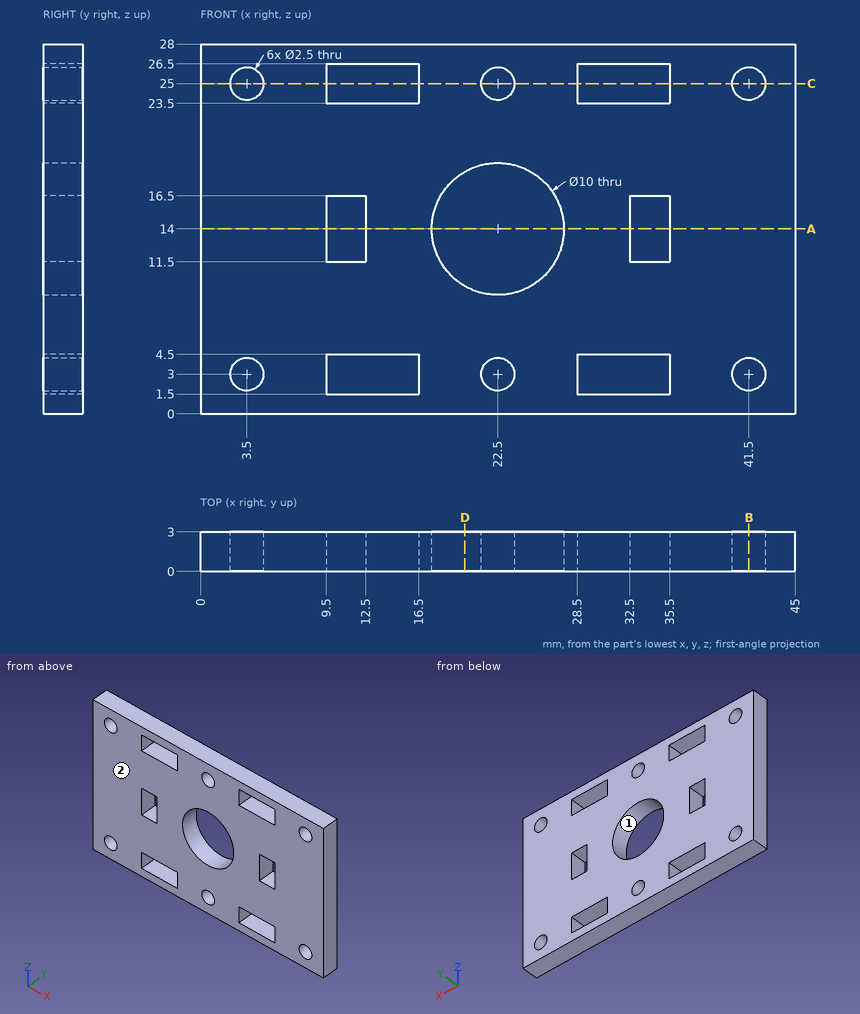
Check sheet for the drawn part. Datum: minimum x, y, z corner. Units: mm. Round coordinates to 2 decimals unless told otherwise and drop trailing zeros. Order: outer loops, then holes, each group sorted by start corner. A loop starts at its lowest first (then second) coordinate and runs counter-clockwise, first axis right, second up. Notation, with made-up numbers: (72, 38.5) -> (111, 38.5) arc R12 cw to (111, 49.5) -> close; hole circle Ø1 at (-22.75, 71.25). An arc over 180 degrees is marked (long way). Put each result on its own line as item: value. Start each with the question number.
(1) Draft check along Z on the marked faces 1 and 2. Enter one of: +Z half, -Z half, draft (parallel to the pull), parting line (faces both ways), or undercut.
(2) Depth check by flat-ended pin: pin 1 Ø3 at (x, z) = (37, 4) entering from -Y. Enter the tip coordinate at first touch or a pass-through.
(3) Section check C-C (z = 25). Enter the section's corners in (x, y), then the cut area to 3 significant figures.
(4) Section check D-D (x = 20). Enter the section's corners in (y, z), then the cut area to 3 significant figures.
(5) Material ranges on line 1 along X through (y, z) = (1.4, 25); line 2 along X through (y, z) = (1.4, 13.75); line 3 along Z through (x, y) = (22.5, 1.6), recorded low to high.
(6) Section check A-A (z = 14). Enter the section's corners in (x, y), then the cut area to 3 significant figures.
(7) Section check B-B (x = 41.5). Enter the section's corners in (y, z).
Completed:
1. face 1: undercut
1. face 2: draft
2. pin 1: stops at y = 0
3. outline: (0, 0) -> (2.25, 0) -> (2.25, 3) -> (0, 3) -> close; (4.75, 0) -> (9.5, 0) -> (9.5, 3) -> (4.75, 3) -> close; (16.5, 0) -> (21.25, 0) -> (21.25, 3) -> (16.5, 3) -> close; (23.75, 0) -> (28.5, 0) -> (28.5, 3) -> (23.75, 3) -> close; (35.5, 0) -> (40.25, 0) -> (40.25, 3) -> (35.5, 3) -> close; (42.75, 0) -> (45, 0) -> (45, 3) -> (42.75, 3) -> close
3. area: 70.5 mm2
4. outline: (0, 0) -> (3, 0) -> (3, 9.67) -> (0, 9.67) -> close; (0, 18.33) -> (3, 18.33) -> (3, 28) -> (0, 28) -> close
4. area: 58.0 mm2
5. line 1: x = 0 to 2.25, 4.75 to 9.5, 16.5 to 21.25, 23.75 to 28.5, 35.5 to 40.25, 42.75 to 45
5. line 2: x = 0 to 9.5, 12.5 to 17.51, 27.49 to 32.5, 35.5 to 45
5. line 3: z = 0 to 1.75, 4.25 to 9, 19 to 23.75, 26.25 to 28
6. outline: (0, 0) -> (9.5, 0) -> (9.5, 3) -> (0, 3) -> close; (12.5, 0) -> (17.5, 0) -> (17.5, 3) -> (12.5, 3) -> close; (27.5, 0) -> (32.5, 0) -> (32.5, 3) -> (27.5, 3) -> close; (35.5, 0) -> (45, 0) -> (45, 3) -> (35.5, 3) -> close
6. area: 87.0 mm2
7. outline: (0, 0) -> (3, 0) -> (3, 1.75) -> (0, 1.75) -> close; (0, 4.25) -> (3, 4.25) -> (3, 23.75) -> (0, 23.75) -> close; (0, 26.25) -> (3, 26.25) -> (3, 28) -> (0, 28) -> close
